Autodesk Inventor part; units mm, degrees
ref_plane "YZ Plane" through (0, 0, 0) normal (1, 0, 0) x (0, 1, 0)
ref_plane "XZ Plane" through (0, 0, 0) normal (0, 1, 0) x (-1, 0, 0)
ref_plane "XY Plane" through (0, 0, 0) normal (0, 0, 1) x (1, 0, 0)
sketch "草图1" plane through (0, 0, 0) normal (0, 1, 0) x (-1, 0, 0)
  line L0 (30.9, 50) -> (30.9, -50)
  line L1 (30.9, -50) -> (-30.9, -50)
  line L2 (-30.9, -50) -> (-30.9, 50)
  line L3 (-30.9, 50) -> (30.9, 50)
  line L4 (0, 0) -> (5.4307, 0)
  line L5 (0, 0) -> (0, 9.1176)
  line L6 (22.9, 42) -> (-22.9, 42)
  line L7 (-22.9, 42) -> (-22.9, -42)
  line L8 (-22.9, -42) -> (22.9, -42)
  line L9 (22.9, -42) -> (22.9, 42)
  circle A0 centre (26.9, 46) radius 1.75
  circle A1 centre (26.9, -46) radius 1.75
  circle A2 centre (-26.9, 46) radius 1.75
  circle A3 centre (-26.9, -46) radius 1.75
  dimension "d0" = 100
  dimension "d1" = 61.8
  dimension "d2" = 8
  dimension "d3" = 8
  dimension "d4" = 3.5
  dimension "d5" = 4
  dimension "d6" = 4
  dimension "d9" = 92
  dimension "d12" = 53.8
extrude "拉伸1" add sketch "草图1" along normal blind 4
sketch "草图2" plane through (0, 4, 0) normal (0, 1, 0) x (1, 0, 0)
  line L0 (-30.9, -50) -> (30.9, -50) construction
  line L1 (-19.2161, -50) -> (-15, -58)
  line L2 (-15, -58) -> (15, -58)
  line L3 (15, -58) -> (19.2161, -50)
  line L4 (0, 0) -> (0, -17.0054)
  line L5 (-19.2161, -50) -> (19.2161, -50)
  dimension "d17" = 8
  dimension "d18" = 30
extrude "拉伸2" add sketch "草图2" against normal blind 3
sketch "草图3" plane through (0, 0, 0) normal (1, 0, 0) x (0, 1, 0)
  line L0 (4, 50) -> (4, 58) construction
  circle A0 centre (4, 54) radius 1.6
  point P0 (0, 0)
  dimension "d21" = 3.2
extrude "拉伸3" cut sketch "草图3" along normal mid plane 40
sketch "草图4" plane through (0, 4, 0) normal (0, 1, 0) x (1, 0, 0)
  line L0 (15, -58) -> (-15, -58) construction
  line L1 (-7, -58) -> (-7, -46)
  line L2 (-7, -46) -> (7, -46)
  line L3 (-30.9, -50) -> (30.9, -50)
  line L4 (7, -46) -> (7, -58)
  line L5 (7, -58) -> (-7, -58)
  line L6 (0, 0) -> (0, -70.1982)
  dimension "d26" = 12
  dimension "d27" = 14
extrude "拉伸4" cut sketch "草图4" against normal blind 40
sketch "草图5" plane through (0, 4, 0) normal (0, 1, 0) x (1, 0, 0)
  circle A0 centre (-26.9, -46) radius 1.75
  circle A1 centre (26.9, 46) radius 1.75
  line L0 (-26.9, -46) -> (26.9, -46)
  line L1 (26.9, -46) -> (26.9, 46)
  line L2 (26.9, 46) -> (-26.9, 46)
  line L3 (-26.9, 46) -> (-26.9, -46)
  point P0 (0, 0)
extrude "拉伸5" cut sketch "草图5" against normal blind 0.5 contours L0 L3 A0 | A0 L3 L2 A1 L1 L0 | A1 L2 L1 picked at (-26.2832, -45.0184) picked at (25.748, 45.8702)
properties part number "筛网"
Read the model definition and answer for the solid it produces. Units are mm, in the model's axes. A direction names the side the tool comes from. Coordinates: 2 decimals unless noted, no trailing zeros. Write each loop counter-clockwise with the first axis right and the second up, starting at its lowest first coordinate (ties: lowest second). Pieces come first, ordered by that corner, then holes. Notation, with made-up numbers: (25.5, -39) -> (41.5, -39) arc R5 ccw to (41.5, -31) -> close; hole circle Ø6 at (70, 45). An arc over 180 degrees is marked (long way). Answer as a JSON object with one key per item and string values.
Q1. The part is cut by section B-B on z = -37. Give the vertices of the cut face in (x, y).
The answers:
{"outline": "(-30.9, 0) -> (-22.9, 0) -> (-22.9, 3.5) -> (-26.9, 3.5) -> (-26.9, 4) -> (-30.9, 4) -> close; (22.9, 0) -> (30.9, 0) -> (30.9, 4) -> (26.9, 4) -> (26.9, 3.5) -> (22.9, 3.5) -> close"}
Q2. Consider line 1 (X direction, y = 0.85, z = -46); line 2 (Z direction, x = 26.9, y = 1.65); line 3 (Z direction, x = 22.5, y = 3.6). Determine where each line is inside the solid, lowest interval first. Write a range as [from, to].
The answers:
{"line 1": "x = [-30.9, -28.65], [-25.15, 25.15], [28.65, 30.9]", "line 2": "z = [-50, -47.75], [-44.25, 44.25], [47.75, 50]", "line 3": "z = [-50, -46], [46, 50]"}
Q3. A tool of negligible diameter and unlimited length cuts with its end or side. For faces 1 (the flat face through (12, 1, 54)), 2 (the flat face through (24, 2, 50)), 3 (the flat face through (-30.9, 2, 1)), 4 (the flat face through (-24, 2, 50)), 5 (the flat face through (22.9, 2, 1)), from which of +Z, -Z, +X, -X, +Y, -Y can it reach the whole face along a straight path? Write none if from no direction.
The answers:
{"face 1": "+Z, +X, -X, -Y", "face 2": "+Z, +X, -Y", "face 3": "+Z, -Z, -X, +Y, -Y", "face 4": "+Z, -X, -Y", "face 5": "+Y, -Y"}
Q4. The part is cut by section C-C on x = 21. Give the vertices of the cut face in (y, z), then the cut area to 3 significant figures.
The answers:
{"outline": "(0, -50) -> (4, -50) -> (4, -46) -> (3.5, -46) -> (3.5, -42) -> (0, -42) -> close; (0, 42) -> (3.5, 42) -> (3.5, 46) -> (4, 46) -> (4, 50) -> (0, 50) -> close", "area": "60.0 mm2"}
Q5. Determine the mould class of faces 6 (the flat face through (0, 2, 46)), 7 (the cylindrical face through (-27.71, 1.97, 47.55)), 8 (the flat face through (-7, 2, 52)) for opening direction Z: pulls with the +Z half, pulls with the -Z half, needs draft (parallel to the pull), parting line crosses it, or undercut.
The answers:
{"face 6": "pulls with the +Z half", "face 7": "undercut", "face 8": "needs draft"}
Q6. The part is cut by section A-A on x = -14. Give the vertices of the cut face in (y, z), then the cut area to 3 significant figures.
The answers:
{"outline": "(0, -50) -> (4, -50) -> (4, -46) -> (3.5, -46) -> (3.5, -42) -> (0, -42) -> close; (0, 42) -> (3.5, 42) -> (3.5, 46) -> (4, 46) -> (4, 52.4) arc R1.6 cw to (4, 55.6) -> (4, 58) -> (1, 58) -> (1, 50) -> (0, 50) -> close", "area": "80.0 mm2"}
Q7. Flat-ended cylindrical pins translate along their axes: pin 1 Ø0.6 at (x, y) = (-6, 3.5) entering from +Z; pin 2 Ø2.5 at (x, z) = (11, 55) entering from -Y. Find the tip coordinate at first contact, or state that the pin passes through.
The answers:
{"pin 1": "stops at z = 46", "pin 2": "stops at y = 1"}
Q8. The part is cut by section D-D on z = 54. Give the vertices of the cut face in (x, y), then the cut area to 3 significant figures.
The answers:
{"outline": "(-17.11, 1) -> (-7, 1) -> (-7, 2.4) -> (-17.11, 2.4) -> close; (7, 1) -> (17.11, 1) -> (17.11, 2.4) -> (7, 2.4) -> close", "area": "28.3 mm2"}
